Here's the drawing with two shaded views (mm, measured from the low corner). I have some questions. Give positions to 0.01 mm unless a question says otherwise; leave off trailing zeros. Loops run counter-clockwise (first coordinate to the right, second up) from the corner with the lowest first, then second, coordinate; pieces in that order, holes last. Notation, with made-up numbers: (72, -39) -> (94, -39) arc R27 cw to (94, -6) -> close; hole circle Ø3 at (-37.5, 72.25). An arc over 180 degrees is marked (long way). Answer in a Markdown table with one row per item. Add a question column.
Item 1: For P1, Ø1.5, axis at y = 1.5, z = 22.5, coming from the -X side; P2, Ø1, axis at x = 65.5, y = 0.5, coming from the -Z side (3 decimals); P3, Ø1.5, axis at y = 2, z = 61.5, coming from the +X side, each with a flat end and sliding along its axis, tell me the tip position at first contact or that it passes through.
Item 2: If we section it at B-B (z = 17.5): Write out the boundary of the cut face in (x, y).
Item 3: If I drill on line 1 (Z direction, x = 11, y = 1.85); line 2 (Z direction, x = 36, y = 2.8); line 3 (X direction, y = 0.8, z = 35), over which ranges is the centre line in solid material (lowest first)?
Item 4: If we section it at C-C (y = 2.2): Write out the boundary of the cut face in (x, z), then the cut area to 3 significant figures.
Item 5: If we section it at A-A (x = 55): Write out the boundary of the cut face in (y, z).
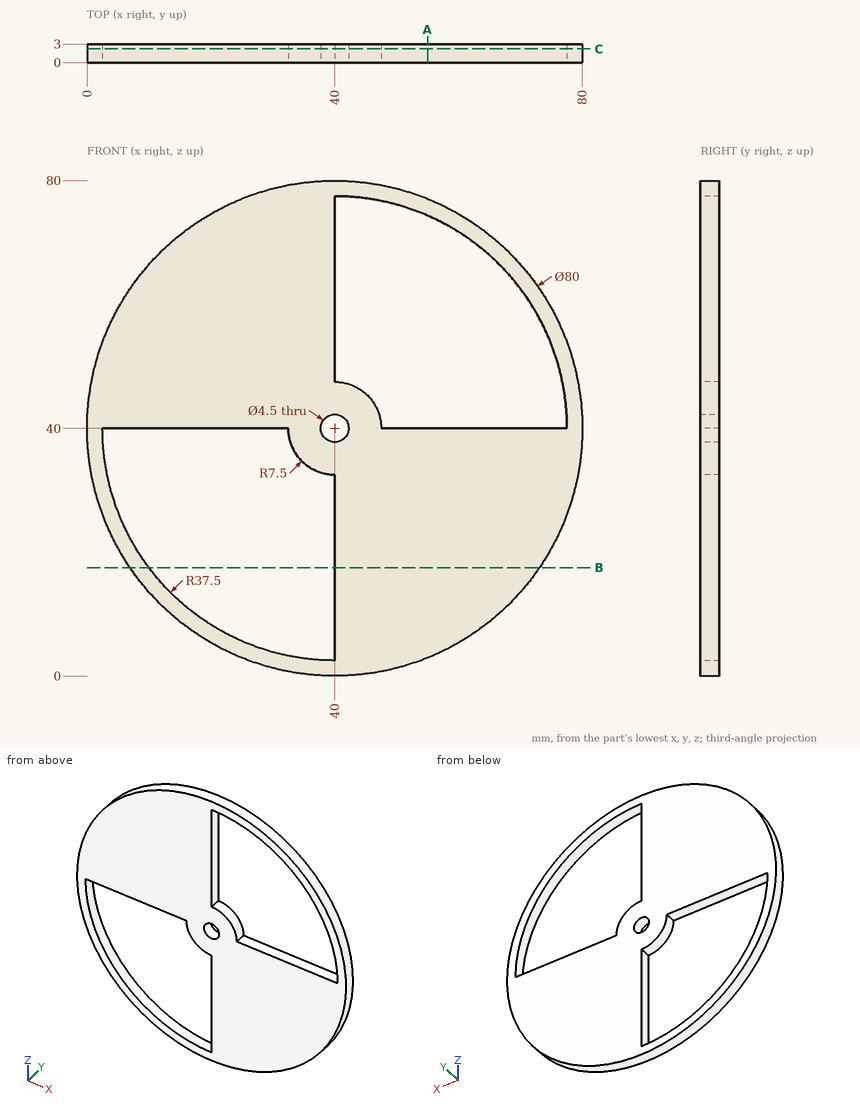
Recorded:
| question | item | result |
|---|---|---|
| 1 | P1 | stops at x = 3.68 |
| 1 | P2 | stops at z = 8.775 |
| 1 | P3 | stops at x = 74.2 |
| 2 | outline | (6.93, 0) -> (10, 0) -> (10, 3) -> (6.93, 3) -> close; (40, 0) -> (73.07, 0) -> (73.07, 3) -> (40, 3) -> close |
| 3 | line 1 | z = 12.45 to 16.23, 40 to 67.55 |
| 3 | line 2 | z = 0.2 to 2.71, 33.66 to 79.8 |
| 3 | line 3 | x = 0.31 to 2.83, 34.41 to 79.69 |
| 4 | outline | circle Ø80 at (40, 40); hole (2.5, 40) arc R37.5 ccw to (40, 2.5) -> (40, 32.5) arc R7.5 cw to (32.5, 40) -> close; hole circle Ø4.5 at (40, 40); hole (40, 47.5) arc R7.5 cw to (47.5, 40) -> (77.5, 40) arc R37.5 ccw to (40, 77.5) -> close |
| 4 | area | 2,890 mm^2 |
| 5 | outline | (0, 2.92) -> (3, 2.92) -> (3, 40) -> (0, 40) -> close; (0, 74.37) -> (3, 74.37) -> (3, 77.08) -> (0, 77.08) -> close |
